Design review of the part built by this model. Coordinates are the model's own, in mm. A direction names the side the tool comes from. Give positions to 0.01 mm unless a question says otherwise; leave off trailing zeros. Answer as a JSON object with one key per item and string values.
Autodesk Inventor part; units mm, degrees
ref_plane "YZ Plane" through (0, 0, 0) normal (1, 0, 0) x (0, 1, 0)
ref_plane "XZ Plane" through (0, 0, 0) normal (0, 1, 0) x (-1, 0, 0)
ref_plane "XY Plane" through (0, 0, 0) normal (0, 0, 1) x (1, 0, 0)
sketch "Sketch1" plane through (0, 0, 0) normal (0, 0, 1) x (1, 0, 0)
  line L0 (0, 0) -> (146, 0)
  line L1 (146, 0) -> (146, 177.5)
  line L2 (146, 177.5) -> (0, 177.5)
  line L3 (0, 177.5) -> (0, 0)
  dimension "d0" = 146
  dimension "d1" = 177.5
extrude "Extrusion1" add sketch "Sketch1" along normal blind 5
sketch "Sketch3" plane through (0, 0, 5) normal (0, 0, 1) x (1, 0, 0)
  line L0 (0, 0) -> (146, 0)
  line L1 (146, 0) -> (146, 177.5)
  line L2 (146, 177.5) -> (0, 177.5)
  line L3 (0, 177.5) -> (0, 0)
  line L4 (0, 141) -> (146, 141) construction
  line L5 (0, 36.5) -> (146, 36.5) construction
  line L6 (22, 177.5) -> (22, 0) construction
  line L7 (81, 0) -> (81, 177.5) construction
  line L8 (140, 177.5) -> (140, 0) construction
  line L9 (20.5, 142.5) -> (23.5, 142.5)
  line L10 (25, 141) -> (25, 141)
  line L11 (23.5, 139.5) -> (20.5, 139.5)
  line L12 (19, 141) -> (19, 141)
  line L13 (19, 142.5) -> (25, 139.5) construction
  line L14 (25, 142.5) -> (19, 139.5) construction
  line L15 (20.5, 38) -> (23.5, 38)
  line L16 (25, 36.5) -> (25, 36.5)
  line L17 (23.5, 35) -> (20.5, 35)
  line L18 (19, 36.5) -> (19, 36.5)
  line L19 (19, 38) -> (25, 35) construction
  line L20 (25, 38) -> (19, 35) construction
  line L21 (138.5, 142.5) -> (141.5, 142.5)
  line L22 (143, 141) -> (143, 141)
  line L23 (141.5, 139.5) -> (138.5, 139.5)
  line L24 (137, 141) -> (137, 141)
  line L25 (137, 142.5) -> (143, 139.5) construction
  line L26 (143, 142.5) -> (137, 139.5) construction
  line L27 (141.5, 38) -> (138.5, 38)
  line L28 (137, 36.5) -> (137, 36.5)
  line L29 (138.5, 35) -> (141.5, 35)
  line L30 (143, 36.5) -> (143, 36.5)
  line L31 (143, 38) -> (137, 35) construction
  line L32 (137, 38) -> (143, 35) construction
  arc A0 (20.5, 142.5) -> (19, 141) centre (20.5, 141) ccw
  arc A1 (25, 141) -> (23.5, 142.5) centre (23.5, 141) ccw
  arc A2 (23.5, 139.5) -> (25, 141) centre (23.5, 141) ccw
  arc A3 (19, 141) -> (20.5, 139.5) centre (20.5, 141) ccw
  arc A4 (20.5, 38) -> (19, 36.5) centre (20.5, 36.5) ccw
  arc A5 (25, 36.5) -> (23.5, 38) centre (23.5, 36.5) ccw
  arc A6 (23.5, 35) -> (25, 36.5) centre (23.5, 36.5) ccw
  arc A7 (19, 36.5) -> (20.5, 35) centre (20.5, 36.5) ccw
  arc A8 (141.5, 35) -> (143, 36.5) centre (141.5, 36.5) ccw
  arc A9 (137, 36.5) -> (138.5, 35) centre (138.5, 36.5) ccw
  arc A10 (138.5, 38) -> (137, 36.5) centre (138.5, 36.5) ccw
  arc A11 (143, 36.5) -> (141.5, 38) centre (141.5, 36.5) ccw
  arc A12 (138.5, 142.5) -> (137, 141) centre (138.5, 141) ccw
  arc A13 (137, 141) -> (138.5, 139.5) centre (138.5, 141) ccw
  arc A14 (143, 141) -> (141.5, 142.5) centre (141.5, 141) ccw
  arc A15 (141.5, 139.5) -> (143, 141) centre (141.5, 141) ccw
  line L33 (69.5, 142.5) -> (92.5, 142.5)
  line L34 (94, 141) -> (94, 141)
  line L35 (92.5, 139.5) -> (69.5, 139.5)
  line L36 (68, 141) -> (68, 141)
  line L37 (68, 142.5) -> (94, 139.5) construction
  line L38 (94, 142.5) -> (68, 139.5) construction
  line L39 (69.5, 38) -> (92.5, 38)
  line L40 (94, 36.5) -> (94, 36.5)
  line L41 (92.5, 35) -> (69.5, 35)
  line L42 (68, 36.5) -> (68, 36.5)
  line L43 (68, 38) -> (94, 35) construction
  line L44 (94, 38) -> (68, 35) construction
  arc A16 (69.5, 142.5) -> (68, 141) centre (69.5, 141) ccw
  arc A17 (68, 141) -> (69.5, 139.5) centre (69.5, 141) ccw
  arc A18 (92.5, 139.5) -> (94, 141) centre (92.5, 141) ccw
  arc A19 (94, 141) -> (92.5, 142.5) centre (92.5, 141) ccw
  arc A20 (69.5, 38) -> (68, 36.5) centre (69.5, 36.5) ccw
  arc A21 (68, 36.5) -> (69.5, 35) centre (69.5, 36.5) ccw
  arc A22 (92.5, 35) -> (94, 36.5) centre (92.5, 36.5) ccw
  arc A23 (94, 36.5) -> (92.5, 38) centre (92.5, 36.5) ccw
  point P0 (22, 141)
  point P1 (22, 36.5)
  point P2 (81, 36.5)
  point P3 (81, 141)
  point P4 (140, 141)
  point P5 (140, 36.5)
  dimension "d22" = 36.5
  dimension "d23" = 36.5
  dimension "d24" = 104.5
  dimension "d25" = 59
  dimension "d26" = 59
  dimension "d36" = 22
  dimension "d39" = 3
  dimension "d40" = 6
  dimension "d41" = 1.5
  dimension "d42" = 1.5
  dimension "d43" = 1.5
  dimension "d44" = 1.5
  dimension "d47" = 26
  dimension "d48" = 26
  dimension "d49" = 3
  dimension "d50" = 3
  dimension "d51" = 1.5
  dimension "d52" = 1.5
extrude "Extrusion4" cut sketch "Sketch3" against normal blind 10 contours L9 A1 A2 L11 A3 A0 | L15 A5 A6 L17 A7 A4 | L21 A14 A15 L23 A13 A12 | A11 A8 L29 A9 A10 L27 | L33 A19 A18 L35 A17 A16 | L39 A23 A22 L41 A21 A20
ref_plane "Work Plane1" through (81, 38, 5) normal (1, 0, 0) x (0, 0, -1)
ref_plane "Work Plane2" through (69.5, 88.75, 5) normal (0, -1, 0) x (1, 0, 0)
properties part number "plate_base" material "Aluminum 6061-AHC"
(1) Tool access review of faces 5 (the flat face through (72, 0, 2)), 6 (the flat face through (81, 142.5, 3)): name each direction out of +Z, -Z, +X, -X, +Y, -Y from which nothing blocks a thin tool from reaching the whole face with its end or side.
Checked values:
{"face 5": "+Z, -Z, +X, -X, -Y", "face 6": "+Z, -Z"}
(2) Draft analysis for pull direction X (two halves, no side actions). For faces 1 (the flat face through (81, 35, 3)), 2 (the flat face through (0, 90, 2)), 3 (the flat face through (81, 38, 3)), 4 (the flat face through (74, 177.5, 2)), state which applies: +X half, -X half, draft (parallel to the pull), parting line (faces both ways), or undercut.
Checked values:
{"face 1": "undercut", "face 2": "-X half", "face 3": "undercut", "face 4": "draft"}
(3) Insertion check: pin 1 (2.5 mm diameter, centred on x = 83.5, z = 3.5, fed in from -Y). The pin has a flat end and moves straight along its axis. Give the tip position at first contact, or say it passes through.
Checked values:
{"pin 1": "stops at y = 0"}
(4) To check wall thickness, follow L1, parallel to X at y = 37.5, z = 3.25; L2, parallel to Y at x = 139.5, z = 3.4. State the ranges of each line that lie inside material, in increasing order. Write a range as from..to.
Checked values:
{"L1": "x = 0..19.38, 24.62..68.38, 93.62..137.38, 142.62..146", "L2": "y = 0..35, 38..139.5, 142.5..177.5"}
